```python
from build123d import *

# Parameters (mm, degrees)
SKETCH1_W                        = 50.8
SKETCH1_H                        = 63.5
BOSS_EXTRUDE1_DEPTH              = 12.7
M8X1_25_TAPPED_HOLE1_D           = 6.8
M8X1_25_TAPPED_HOLE1_DEPTH       = 15
M8X1_25_TAPPED_HOLE1_CSINK_D     = 8.05
M8X1_25_TAPPED_HOLE1_CSINK_ANGLE = 90
M8X1_25_TAPPED_HOLE1_TIP         = 2.042926105
M8X1_25_TAPPED_HOLE2_D           = 6.8
M8X1_25_TAPPED_HOLE2_DEPTH       = 15
M8X1_25_TAPPED_HOLE2_CSINK_D     = 8.05
M8X1_25_TAPPED_HOLE2_CSINK_ANGLE = 90
M8X1_25_TAPPED_HOLE2_TIP         = 2.042926105
CUT_EXTRUDE1_DEPTH               = 13.7


with BuildPart() as part:
    # Sketch1 → Boss-Extrude1 (new body)
    with BuildSketch(Plane(origin=(0, 0, 0), x_dir=(1, 0, 0), z_dir=(0, 1, 0))):
        with Locations((25.4, 31.75)):
            Rectangle(SKETCH1_W, SKETCH1_H)
    extrude(amount=BOSS_EXTRUDE1_DEPTH)

    # M8x1.25 Tapped Hole1
    with Locations(Plane(origin=(0, 0, -63.5), x_dir=(-1, 0, 0), z_dir=(0, 0, -1))):
        with Locations((-25.4, 6.35)):
            CounterSinkHole(M8X1_25_TAPPED_HOLE1_D / 2, M8X1_25_TAPPED_HOLE1_CSINK_D / 2, depth=M8X1_25_TAPPED_HOLE1_DEPTH, counter_sink_angle=M8X1_25_TAPPED_HOLE1_CSINK_ANGLE)
            with Locations((0, 0, -(M8X1_25_TAPPED_HOLE1_DEPTH + M8X1_25_TAPPED_HOLE1_TIP / 2))):  # 118° drill point
                Cone(0, M8X1_25_TAPPED_HOLE1_D / 2, M8X1_25_TAPPED_HOLE1_TIP, mode=Mode.SUBTRACT)

    # M8x1.25 Tapped Hole2
    with Locations(Plane.XY):
        with Locations((25.4, 6.35)):
            CounterSinkHole(M8X1_25_TAPPED_HOLE2_D / 2, M8X1_25_TAPPED_HOLE2_CSINK_D / 2, depth=M8X1_25_TAPPED_HOLE2_DEPTH, counter_sink_angle=M8X1_25_TAPPED_HOLE2_CSINK_ANGLE)
            with Locations((0, 0, -(M8X1_25_TAPPED_HOLE2_DEPTH + M8X1_25_TAPPED_HOLE2_TIP / 2))):  # 118° drill point
                Cone(0, M8X1_25_TAPPED_HOLE2_D / 2, M8X1_25_TAPPED_HOLE2_TIP, mode=Mode.SUBTRACT)

    # Sketch9 → Cut-Extrude1 (cut, through all)
    with BuildSketch(Plane(origin=(0, 12.7, 0), x_dir=(1, 0, 0), z_dir=(0, 1, 0))):
        with BuildLine():
            Line((0, 53.5), (40.8, 53.5))
            ThreePointArc((40.8, 53.5), (44.8, 49.5), (40.8, 45.5))
            Line((40.8, 45.5), (0, 45.5))
            Line((0, 45.5), (0, 53.5))
        make_face()
        with BuildLine():
            Line((50.8, 18), (10, 18))
            ThreePointArc((10, 18), (6, 14), (10, 10))
            Line((10, 10), (50.8, 10))
            Line((50.8, 10), (50.8, 18))
        make_face()
    extrude(amount=-CUT_EXTRUDE1_DEPTH, mode=Mode.SUBTRACT)


solid = part.part
```
Geometry: final body of the model. Coordinates: model frame, mm. A direction names the side the tool comes from. Round coordinates to 2 decimals unless told otherwise and drop trailing zeros. Order: outer loops, then holes, each group sorted by start corner. A loop starts at its lowest first (then second) coordinate and runs counter-clockwise, first axis right, second up. Notation, with made-up numbers: M -28,-1.5 L -16,-1.5 A29 ccw -16,29.5 Z; hole C 35,-30.5 d2. An arc over 180 degrees is marked long. Use one line per item in the form item = value. Start each with the question number.
Q1. Access query for faces 1 (the face through (26.14, 3.03, -5.38)), 2 (the face through (30, 6, -10)), 3 (the face through (22.702, 4.281, -58.122)). Directions: +Z, -Z, +X, -X, +Y, -Y. A direction counts if a zero-diameter tool reaches every point of the face in a straight line with its end or side. Return the directions, or none.
Q2. Material intervals for line 1 (Z direction, x = 36.5, y = 7.25); line 2 (X direction, y = 6.35, z = -55.5); line 3 (Y direction, x = 25.4, z = -57.75), sorted ascending. Write a range as [from, to].
Q3. Cut plane D-D (x = 25.4). Return loops of the section in (y, z) (3 decimals), and give its area (3 significant figures).
Q4. Cut plane C-C (x = 33). Return loops of the section in (y, z).
Q5. Cut plane A-A (y = 6.35). Return loops of the section in (x, z) (3 decimals).
Q6. Mould query, pull axis Z, two halves, no side actions, for faces 4 (the face through (31, 6, -18)), 5 (the face through (0, 6, -22)), 6 (the face through (25, 2, -63.5)). Classes: +Z half, -Z half, draft (parallel to the pull), parting line (faces both ways), or undercut.
Q7. Cut plane B-B (x = 46.5). Return loops of the section in (y, z), and give its area (3 significant figures).
Geometry results:
q1.face_1 = +Z
q1.face_2 = +X, +Y, -Y
q1.face_3 = -Z
q2.line_1 = [-63.5, -53.5], [-45.5, -18], [-10, 0]
q2.line_2 = [0, 22], [28.8, 50.8]
q2.line_3 = [0, 2.95], [9.75, 12.7]
q3.outline = M 0,-63.5 L 2.325,-63.5 L 2.95,-62.875 L 2.95,-53.5 L 0,-53.5 Z; M 0,-45.5 L 12.7,-45.5 L 12.7,-18 L 0,-18 Z; M 0,-10 L 2.95,-10 L 2.95,-0.625 L 2.325,0 L 0,0 Z; M 9.75,-62.875 L 10.375,-63.5 L 12.7,-63.5 L 12.7,-53.5 L 9.75,-53.5 Z; M 9.75,-10 L 12.7,-10 L 12.7,0 L 10.375,0 L 9.75,-0.625 Z
q3.area = 466 mm^2
q4.outline = M 0,-63.5 L 12.7,-63.5 L 12.7,-53.5 L 0,-53.5 Z; M 0,-45.5 L 12.7,-45.5 L 12.7,-18 L 0,-18 Z; M 0,-10 L 12.7,-10 L 12.7,0 L 0,0 Z
q5.outline = M 0,-63.5 L 21.375,-63.5 L 22,-62.875 L 22,-53.5 L 0,-53.5 Z; M 0,-45.5 L 40.8,-45.5 A4 cw 40.8,-53.5 L 28.8,-53.5 L 28.8,-62.875 L 29.425,-63.5 L 50.8,-63.5 L 50.8,-18 L 10,-18 A4 cw 10,-10 L 22,-10 L 22,-0.625 L 21.375,0 L 0,0 Z; M 28.8,-10 L 50.8,-10 L 50.8,0 L 29.425,0 L 28.8,-0.625 Z
q6.face_4 = undercut
q6.face_5 = draft
q6.face_6 = -Z half
q7.outline = M 0,-63.5 L 12.7,-63.5 L 12.7,-18 L 0,-18 Z; M 0,-10 L 12.7,-10 L 12.7,0 L 0,0 Z
q7.area = 705 mm^2
